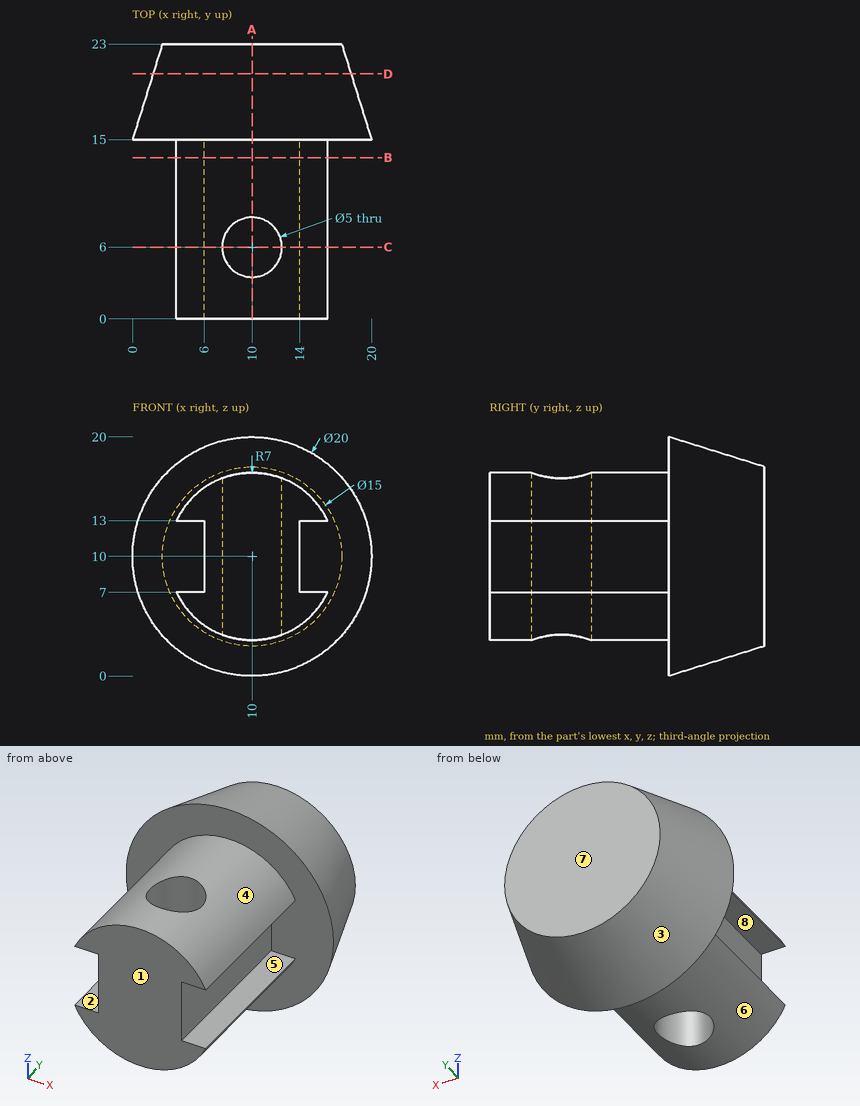
Part print with two shaded views. Sizes in mm from the minimum x, y, z corner. A direction names the side the tool comes from. Round coordinates to 2 decimals unless told otherwise and drop trailing zeros. Order: outer loops, then holes, each group sorted by start corner. A loop starts at its lowest first (then second) coordinate and runs counter-clockwise, first axis right, second up. Notation, with made-up numbers: (56.5, 53) - (64.5, 53) arc R14 cw to (64.5, 59) - close; hole circle Ø10 at (21, 34.25). An arc over 180 degrees is marked (long way). Answer in a Markdown table with one row per item. Add a question column.
(1) Drop flat-ended pins along their axis: pin 1 Ø2 at (x, y) = (2.5, 14.5) entering from -Z; pin 2 Ø0.7 at (x, y) = (5, 7.5) entering from +Z; pin 3 Ø1.2 at (x, y) = (15, 10) entering from -Z. Give the stop position or say it passes through.
(2) Band-saw the part on A-A on x = 10. List the corners of the cut face in (y, z), and give its area (3 significant figures).
(3) Band-saw the part on D-D on y = 20.5. List the corners of the cut face in (x, z).
(4) Band-saw the part on B-B on y = 13.5. List the corners of the cut face in (x, z), and give its area (3 significant figures).
(5) Probe L1, parallel to Y at x = 10, z = 12.75; L2, parallel to Y at x = 14.75, z = 10.5; L3, parallel to X at y = 11, z = 11.25. List the from-to ranges inside material, lowest first. Write a range as [from, to].
(6) Mould opens along Z. For the marked faces 1, 2 and 3 say: +Z half, -Z half, draft (parallel to the pull), parting line (faces both ways), or undercut.
(7) 3-axis set-ups, long thin cutter, end or side, ignore diameter. For the marked faces 4, 5, 6, 7 and 8: which of +Z, -Z, +X, -X, +Y, -Y reach the whole face in a straight line?
(8) Band-saw the part on C-C on y = 6. List the corners of the cut face in (x, z), and give its area (3 significant figures).
Data:
| question | item | result |
|---|---|---|
| 1 | pin 1 | stops at z = 2.52 |
| 1 | pin 2 | stops at z = 15.23 |
| 1 | pin 3 | stops at z = 4.56 |
| 2 | outline | (0, 3) - (3.5, 3) - (3.5, 17) - (0, 17) - close; (8.5, 3) - (15, 3) - (15, 0) - (23, 2.5) - (23, 17.5) - (15, 20) - (15, 17) - (8.5, 17) - close |
| 2 | area | 280 mm^2 |
| 3 | outline | circle Ø16.56 at (10, 10) |
| 4 | outline | (3.68, 7) arc R7 ccw to (16.32, 7) - (14, 7) - (14, 13) - (16.32, 13) arc R7 ccw to (3.68, 13) - (6, 13) - (6, 7) - close |
| 4 | area | 121 mm^2 |
| 5 | L1 | y = [0, 3.5], [8.5, 23] |
| 5 | L2 | y = [15, 23] |
| 5 | L3 | x = [6, 14] |
| 6 | face 1 | draft |
| 6 | face 2 | undercut |
| 6 | face 3 | parting line |
| 7 | face 4 | +Z, -Y |
| 7 | face 5 | +X, -Y |
| 7 | face 6 | -Z, -Y |
| 7 | face 7 | +Z, -Z, +X, -X, +Y |
| 7 | face 8 | -X, -Y |
| 8 | outline | (3.68, 7) arc R7 ccw to (7.5, 3.46) - (7.5, 16.54) arc R7 ccw to (3.68, 13) - (6, 13) - (6, 7) - close; (12.5, 3.46) arc R7 ccw to (16.32, 7) - (14, 7) - (14, 13) - (16.32, 13) arc R7 ccw to (12.5, 16.54) - close |
| 8 | area | 52.1 mm^2 |
